Geometry: see drawing. Coordinates: mm, zero at the bounding-box minimum. A direction names the side the tool comes from. Round coordinates to 2 decimals unless told otherwise and drop trailing zeros. Order: outer loops, then holes, each group sorted by start corner. A loop starts at its lowest first (then second) coordinate and runs counter-clockwise, first axis right, second up. Notation, with made-up numbers: (-30.5, 73) - (11.5, 73) arc R21 ccw to (11.5, 99) - close; hole circle Ø9 at (27.5, 0.25). An arc over 180 degrees is marked (long way). Put each result on its own line as item: value. Start each with the question number.
1) Section D-D on z = 21.5. Output: boundary loops of the cut face in (x, y).
2) Section C-C on x = 18.6. Output: boundary loops of the cut face in (y, z), then the cut area to 3 significant figures.
3) Access query for the marked faces 4 and 5. Directions: +Z, -Z, +X, -X, +Y, -Y. A direction counts if a zero-diameter tool reaches every point of the face in a straight line with its end or side. Return the directions, or none.
4) Section B-B on y = 29. Output: boundary loops of the cut face in (x, z), then the cut area to 3 significant figures.
5) Line query: probe 1 along X at (y, z) = (7.5, 16.5); probe 2 along Z at (x, y) = (0.4, 46.6); probe 3 along Y at (x, z) = (18.5, 9.25). Output: solid intervals per line, ascending. Write a range as [from, to].
6) Contact query for a flat-ended pin moving along its axis: P1, Ø13.5, axis at x = 38, z = 11, coming from the +Y side. Output: stop coordinate, or through.
7) Mould query, pull axis X, two halves, no side actions, for the marked faces 1, 2 and 3. Classes: +X half, -X half, draft (parallel to the pull), parting line (faces both ways), or undercut.
8) Section A-A on y = 38.6. Output: boundary loops of the cut face in (x, z).
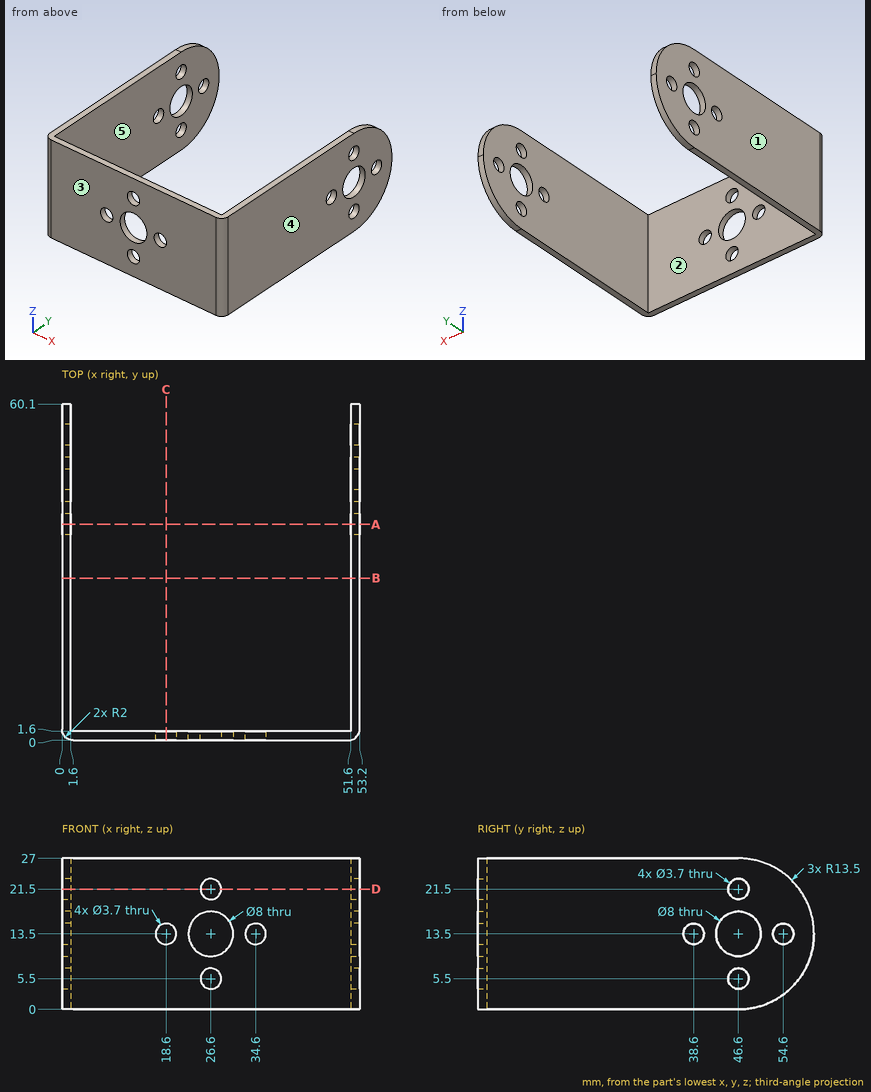
Answer sheet:
1. outline: (0, 2) arc R2 ccw to (2, 0) - (24.75, 0) - (24.75, 1.6) - (1.6, 1.6) - (1.6, 44.75) - (0, 44.75) - close; (0, 48.45) - (1.6, 48.45) - (1.6, 57.47) - (0, 57.47) - close; (28.45, 0) - (51.2, 0) arc R2 ccw to (53.2, 2) - (53.2, 44.75) - (51.6, 44.75) - (51.6, 1.6) - (28.45, 1.6) - close; (51.6, 48.45) - (53.2, 48.45) - (53.2, 57.47) - (51.6, 57.47) - close
2. outline: (0, 0) - (1.6, 0) - (1.6, 11.65) - (0, 11.65) - close; (0, 15.35) - (1.6, 15.35) - (1.6, 27) - (0, 27) - close
2. area: 37.3 mm^2
3. face 4: +Z, -Z, +X, +Y, -Y
3. face 5: +Z, -Z, +Y
4. outline: (0, 0) - (1.6, 0) - (1.6, 27) - (0, 27) - close; (51.6, 0) - (53.2, 0) - (53.2, 27) - (51.6, 27) - close
4. area: 86.4 mm^2
5. probe 1: [0, 1.6], [51.6, 53.2]
5. probe 2: [0, 3.65], [7.35, 9.5], [17.5, 19.65], [23.35, 27]
5. probe 3: [0, 1.6]
6. P1: y = 1.6
7. face 1: -X half
7. face 2: undercut
7. face 3: draft
8. outline: (0, 0) - (1.6, 0) - (1.6, 11.65) - (0, 11.65) - close; (0, 15.35) - (1.6, 15.35) - (1.6, 27) - (0, 27) - close; (51.6, 0) - (53.2, 0) - (53.2, 11.65) - (51.6, 11.65) - close; (51.6, 15.35) - (53.2, 15.35) - (53.2, 27) - (51.6, 27) - close
